from build123d import *

# Parameters (mm, degrees)
SKETCH1_R           = 13
SKETCH1_R_2         = 7
BOSS_EXTRUDE1_DEPTH = 62
FILLET2_R           = 1
FILLET3_R           = 1


with BuildPart() as part:
    # Sketch1 → Boss-Extrude1 (new body)
    with BuildSketch(Plane(origin=(0, 0, 0), x_dir=(1, 0, 0), z_dir=(0, 1, 0))):
        with Locations(Location((0, 0, 0), (0, 0, 270))):
            Circle(SKETCH1_R)
        with Locations(Location((0, 0, 0), (0, 0, 270))):
            Circle(SKETCH1_R_2, mode=Mode.SUBTRACT)
    extrude(amount=BOSS_EXTRUDE1_DEPTH)

    # Fillet2
    fillet2_edges = [part.edges().sort_by_distance(p)[0] for p in [
        (0, 0, -13),
        (0, 62, -13),
    ]]
    fillet(fillet2_edges, radius=FILLET2_R)

    # Fillet3
    fillet3_edges = [part.edges().sort_by_distance(p)[0] for p in [
        (0, 0, -7),
        (0, 62, -7),
    ]]
    fillet(fillet3_edges, radius=FILLET3_R)


solid = part.part
For this review, take the finished solid that the model builds, in its own axes (mm). Round coordinates to 2 decimals unless told otherwise and drop trailing zeros. Write each loop counter-clockwise with the first axis right and the second up, starting at its lowest first coordinate (ties: lowest second). Pieces come first, ordered by that corner, then holes. Notation, with made-up numbers: (27.25, -20) - (37.25, -20) arc R26 ccw to (37.25, 0) - close; hole circle Ø1 at (40.25, 85). An arc over 180 degrees is marked (long way). Write item = value, one per line. Start each with the question number.
1. Consider section C-C on y = 56. State the section outline as (x, z) points.
2. For pin 1 Ø6 at (y, z) = (37, -3.5) entering from +X; pin 2 Ø6 at (x, y) = (-2, 8) entering from -Z; pin 3 Ø4 at (y, z) = (7.5, -9) entering from +X; pin 4 Ø6 at (y, z) = (19.5, 9) entering from +X, all flat-tipped, find the tip position at first contact; note any pin that passes through.
3. Consider section B-B on z = 0. State the section outline as (x, y) points.
4. Draft analysis for pull direction Z (two halves, no side actions). For faces 1 (the face through (-6.834, 30.58, -1.517)), 2 (the face through (-8, 62, 2)), 3 (the face through (-7.91, 30.58, -10.316)), state which applies: released by +Z, released by -Z, zero draft, split by the parting line, or undercut.
5. Consider section A-A on x = 0. State the section outline as (y, z) points.
6. Wall thickness on L1, parallel to X at y = 34, z = 0; L2, parallel to Z at x = -2, y = 43; L3, parallel to Z at x = -6, y = 18.5: over which ranges is each line inside the solid? List them lowest first.
Evaluation:
q1.outline = circle Ø26 at (0, 0); hole circle Ø14 at (0, 0)
q2.pin_1 = 12.99
q2.pin_2 = -13
q2.pin_3 = 10.95
q2.pin_4 = 11.53
q3.outline = (-13, 1) arc R1 ccw to (-12, 0) - (-8, 0) arc R1 ccw to (-7, 1) - (-7, 61) arc R1 ccw to (-8, 62) - (-12, 62) arc R1 ccw to (-13, 61) - close; (7, 1) arc R1 ccw to (8, 0) - (12, 0) arc R1 ccw to (13, 1) - (13, 61) arc R1 ccw to (12, 62) - (8, 62) arc R1 ccw to (7, 61) - close
q4.face_1 = undercut
q4.face_2 = zero draft
q4.face_3 = split by the parting line
q5.outline = (0, -12) arc R1 ccw to (1, -13) - (61, -13) arc R1 ccw to (62, -12) - (62, -8) arc R1 ccw to (61, -7) - (1, -7) arc R1 ccw to (0, -8) - close; (0, 8) arc R1 ccw to (1, 7) - (61, 7) arc R1 ccw to (62, 8) - (62, 12) arc R1 ccw to (61, 13) - (1, 13) arc R1 ccw to (0, 12) - close
q6.L1 = -13 to -7, 7 to 13
q6.L2 = -12.85 to -6.71, 6.71 to 12.85
q6.L3 = -11.53 to -3.61, 3.61 to 11.53
